Work out the finished part from the listing and answer in its coordinate system (mm). A direction names the side the tool comes from. Coordinates: 2 decimals unless noted, no trailing zeros. Order: outer loops, then holes, each group sorted by start corner. A loop starts at its lowest first (then second) coordinate and runs counter-clockwise, first axis right, second up. Notation, with made-up numbers: (19.25, -25.5) -> (34.25, -25.5) arc R16 ccw to (34.25, 4.5) -> close; hole circle Ø5 at (-11.5, 15). An arc over 180 degrees is marked (long way). Use one line per item in the form item = value.
from build123d import *

# Parameters (mm, degrees)
F0_R     = 3.81
F1_DEPTH = 6.35
F2_R     = 8.7376
F3_DEPTH = 6.35
F4_R     = 5.08


with BuildPart() as f1:
    # F0 (on Front) → F1 (new body)
    with BuildSketch(Plane.XZ):
        Polygon((19.05, 7.890768), (7.890768, 19.05), (-7.890768, 19.05), (-19.05, 7.890768), (-19.05, -7.890768), (-7.890768, -19.05), (7.890768, -19.05), (19.05, -7.890768), align=None)
        Circle(F0_R, mode=Mode.SUBTRACT)
    extrude(amount=F1_DEPTH)

    # F2 (on face) → F3 (join)
    with BuildSketch(Plane.XZ.offset(6.35)):
        Circle(F2_R)
        Polygon((-3.204236, -5.5499), (-6.408473, 0), (-3.204236, 5.5499), (3.204236, 5.5499), (6.408473, 0), (3.204236, -5.5499), align=None, mode=Mode.SUBTRACT)
    extrude(amount=F3_DEPTH)

    # F4
    f4_edges = [f1.edges().sort_by_distance(p)[0] for p in [
        (7.890768, -3.175, 19.05),
        (19.05, -3.175, 7.890768),
        (19.05, -3.175, -7.890768),
        (7.890768, -3.175, -19.05),
        (-7.890768, -3.175, -19.05),
        (-19.05, -3.175, -7.890768),
        (-19.05, -3.175, 7.890768),
        (-7.890768, -3.175, 19.05),
    ]]
    fillet(f4_edges, radius=F4_R)


solid = f1.part
(1) Straight lines are drawn through the part: line 1 along Z through (x, y) = (0, -4.25); line 2 along Y through (x, z) = (-3.5, -3.5); line 3 along Z through (x, y) = (2, -8.5). For each, find the intervals that lie inside material, in ascending order.
Data:
line_1 = -19.05 to -3.81, 3.81 to 19.05
line_2 = -6.35 to 0
line_3 = -8.51 to -5.55, 5.55 to 8.51
(2) Section A-A on y = -1.25 is taken. Write down the section's boundary in (x, z), plus the area to 3 significant figures.
Data:
outline = (-19.05, -5.79) arc R5.08 ccw to (-17.56, -9.38) -> (-9.38, -17.56) arc R5.08 ccw to (-5.79, -19.05) -> (5.79, -19.05) arc R5.08 ccw to (9.38, -17.56) -> (17.56, -9.38) arc R5.08 ccw to (19.05, -5.79) -> (19.05, 5.79) arc R5.08 ccw to (17.56, 9.38) -> (9.38, 17.56) arc R5.08 ccw to (5.79, 19.05) -> (-5.79, 19.05) arc R5.08 ccw to (-9.38, 17.56) -> (-17.56, 9.38) arc R5.08 ccw to (-19.05, 5.79) -> close; hole circle Ø7.62 at (0, 0)
area = 1,150 mm²
(3) Each of these flat-tipped pins is pushed along its axis until it touches: P1, Ø2, axis at y = -10.5, z = 5, coming from the +X side; P2, Ø1, axis at x = -12.5, y = -5.5, coming from the -Z side. Where does it stop, or does it pass through?
Data:
P1 = 7.77
P2 = -14.94
(4) Section C-C on y = -7 is taken. Write down the section's boundary in (x, z).
Data:
outline = circle Ø17.48 at (0, 0); hole (-6.41, 0) -> (-3.2, -5.55) -> (3.2, -5.55) -> (6.41, 0) -> (3.2, 5.55) -> (-3.2, 5.55) -> close
(5) Section D-D on x = -4.5 is taken. Write down the section's boundary in (y, z).
Data:
outline = (-12.7, -7.49) -> (-6.35, -7.49) -> (-6.35, -19.05) -> (0, -19.05) -> (0, 19.05) -> (-6.35, 19.05) -> (-6.35, 7.49) -> (-12.7, 7.49) -> (-12.7, 3.31) -> (-6.35, 3.31) -> (-6.35, -3.31) -> (-12.7, -3.31) -> close
(6) Section B-B on x = 0 is taken. Write down the section's boundary in (y, z).
Data:
outline = (-12.7, -8.74) -> (-6.35, -8.74) -> (-6.35, -19.05) -> (0, -19.05) -> (0, -3.81) -> (-6.35, -3.81) -> (-6.35, -5.55) -> (-12.7, -5.55) -> close; (-12.7, 5.55) -> (-6.35, 5.55) -> (-6.35, 3.81) -> (0, 3.81) -> (0, 19.05) -> (-6.35, 19.05) -> (-6.35, 8.74) -> (-12.7, 8.74) -> close
(7) The mould has two halves that part along X. Classify faces 1 (the flat face through (-13.41, -3.13, 13.53)), 2 (the flat face through (1, -6.35, 4)), 3 (the flat face through (0, -9, 5.55)), 4 (the cylindrical face through (18.674, -3.219, -7.705)): released by +X, released by -X, zero draft, split by the parting line, or undercut.
Data:
face_1 = released by -X
face_2 = undercut
face_3 = undercut
face_4 = released by +X
(8) Which of the six approach directions +Z, -Z, +X, -X, +Y, -Y give full straight-line access (tool end or side, diameter ignored) to faces 5 (the flat face through (0, -3, -19.05)), 6 (the cylindrical face through (8.334, -9.481, 2.625))?
Data:
face_5 = -Z, +X, -X, +Y, -Y
face_6 = -Y
